Verification items for the finished model (mm, model axes). Face numbers are marked on the shaded views. A direction names the side the tool comes from. Coordinates: 2 decimals unless noted, no trailing zeros. Write each loop counter-clockwise with the first axis right and the second up, starting at its lowest first coordinate (ties: lowest second). Pieces come first, ordered by that corner, then holes. Notation, with made-up numbers: (19, 11) -> (48, 11) arc R23 cw to (48, 29) -> close; hole circle Ø4 at (-5.5, 72.25). An arc over 180 degrees is marked (long way). Answer in a Markdown table with one row per item.
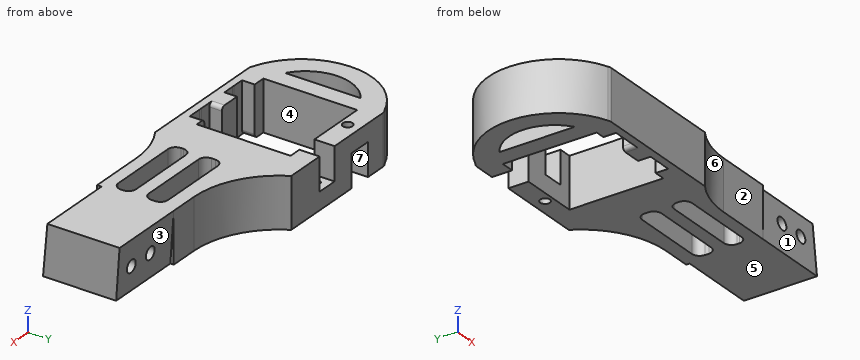
```python
from build123d import *

# Parameters (mm, degrees)
SKETCH_1_W           = 32.6
SKETCH_1_H           = 34.6
SKETCH_1_R           = 1.25
SKETCH_1_W_2         = 24.6
SKETCH_1_H_2         = 24.2
EXTRUDE_1_DEPTH      = 13
SKETCH_3_W           = 6.5
SKETCH_3_H           = 6.519005167
CUT_EXTRUDE_1_DEPTH  = 19
SKETCH_4_W           = 6.5
SKETCH_4_H           = 6.467668889
CUT_EXTRUDE_2_DEPTH  = 23
EXTRUDE_2_DEPTH      = 50
SKETCH_1_2_W         = 22.27659965
SKETCH_1_2_H         = 4.598586669
SKETCH_1_2_W_2       = 22.283050596
SKETCH_1_2_H_2       = 4.977540741
CUT_EXTRUDE_5_DEPTH  = 34
FILLET_1_R           = 2
FILLET_2_R           = 2
FILLET_5_R           = 1
SKETCH_9_W           = 54.594998093
SKETCH_9_H           = 18.111982385
SKETCH_9_W_2         = 52.534809486
SKETCH_9_H_2         = 12.989301534
CUT_EXTRUDE_6_DEPTH  = 41
FILLET_6_R           = 22
EXTRUDE_4_DEPTH      = 13
SKETCH_13_W          = 5.518907879
SKETCH_13_H          = 8.361822047
CUT_EXTRUDE_8_DEPTH  = 8.5
SKETCH_14_W          = 6.038657432
SKETCH_14_H          = 7.741248121
CUT_EXTRUDE_9_DEPTH  = 8.5
SKETCH_15_OUTSIDE_W  = 35.102
SKETCH_15_OUTSIDE_H  = 56.702
CUT_EXTRUDE_11_DEPTH = 20
SKETCH_20_R          = 1.625
CUT_EXTRUDE_15_DEPTH = 40


with BuildPart() as part:
    # Sketch 1 → 凸台-拉伸1 (new body)
    with BuildSketch(Plane.XY):
        with Locations((-9.850980392, 1.274712581)):
            Rectangle(SKETCH_1_W, SKETCH_1_H)
        with Locations(Location((-15.700980392, 15.424712581, 0), (0, 0, 180))):
            Circle(SKETCH_1_R, mode=Mode.SUBTRACT)
        with Locations(Location((-3.600980392, 15.424712581, 0), (0, 0, 180))):
            Circle(SKETCH_1_R, mode=Mode.SUBTRACT)
        with Locations(Location((-15.700980392, -12.875287419, 0), (0, 0, 180))):
            Circle(SKETCH_1_R, mode=Mode.SUBTRACT)
        with Locations(Location((-3.600980392, -12.875287419, 0), (0, 0, 180))):
            Circle(SKETCH_1_R, mode=Mode.SUBTRACT)
        with Locations((-9.850980392, 1.274712581)):
            Rectangle(SKETCH_1_W_2, SKETCH_1_H_2, mode=Mode.SUBTRACT)
    extrude(amount=EXTRUDE_1_DEPTH)

    # 草图3 → 切除-拉伸1 (cut)
    with BuildSketch(Plane(origin=(0, 0, 0), x_dir=(-1, 0, 0), z_dir=(0, 0, -1))):
        with Locations((15.700980392, -10.82528742)):
            Rectangle(SKETCH_3_W, SKETCH_3_H)
    extrude(amount=-CUT_EXTRUDE_1_DEPTH, mode=Mode.SUBTRACT)

    # 草图4 → 切除-拉伸2 (cut)
    with BuildSketch(Plane.XY.offset(13)):
        with Locations((-3.600980392, -10.82528742)):
            Rectangle(SKETCH_4_W, SKETCH_4_H)
    extrude(amount=-CUT_EXTRUDE_2_DEPTH, mode=Mode.SUBTRACT)

    # 草图5 → 凸台-拉伸2 (add)
    with BuildSketch(Plane(origin=(6.449019608, 0, 0), x_dir=(0, 0, -1), z_dir=(1, 0, 0))):
        Polygon((-13, 18.574712581), (-13, 10.055461473), (-13, -16.025287419), (0, -16.025287419), (0, -15.027567927), (0, 16.282461831), (0, 18.574712581), align=None)
    extrude(amount=EXTRUDE_2_DEPTH)

    # Sketch 1 2 → 切除-拉伸5 (cut)
    with BuildSketch(Plane.XY.offset(13)):
        with Locations((24.037173058, -7.263594431)):
            Rectangle(SKETCH_1_2_W, SKETCH_1_2_H)
        with Locations((24.078382453, 0.81654228)):
            Rectangle(SKETCH_1_2_W_2, SKETCH_1_2_H_2)
    extrude(amount=-CUT_EXTRUDE_5_DEPTH, mode=Mode.SUBTRACT)

    # 圆角1
    fillet_1_edges = [part.edges().sort_by_distance(p)[0] for p in [
        (12.936857155, -1.672228091, 6.5),
        (12.936857155, 3.30531265, 6.5),
        (35.219907751, 3.30531265, 6.5),
        (35.219907751, -1.672228091, 6.5),
        (12.898873233, -9.562887765, 6.5),
        (12.898873233, -4.964301096, 6.5),
        (35.175472883, -4.964301096, 6.5),
        (35.175472883, -9.562887765, 6.5),
    ]]
    fillet(fillet_1_edges, radius=FILLET_1_R)

    # 圆角2
    fillet_2_edges = [part.edges().sort_by_distance(p)[0] for p in [
        (-26.150980392, -16.025287419, 6.5),
        (-26.150980392, 18.574712581, 6.5),
    ]]
    fillet(fillet_2_edges, radius=FILLET_2_R)

    # 圆角5
    fillet_5_edges = [part.edges().sort_by_distance(p)[0] for p in [
        (-12.450980392, -12.455038711, 0),
        (-18.950980392, -12.455038711, 0),
        (-6.850980392, -12.442204642, 13),
        (-0.350980392, -12.442204642, 13),
    ]]
    fillet(fillet_5_edges, radius=FILLET_5_R)

    # 草图9 → 切除-拉伸6 (cut)
    with BuildSketch(Plane(origin=(0, 0, 0), x_dir=(-1, 0, 0), z_dir=(0, 0, -1))):
        with Locations((-36.934177516, 16.051357777)):
            Rectangle(SKETCH_9_W, SKETCH_9_H)
        with Locations((-36.653242706, -19.247200889)):
            Rectangle(SKETCH_9_W_2, SKETCH_9_H_2)
    extrude(amount=-CUT_EXTRUDE_6_DEPTH, mode=Mode.SUBTRACT)

    # 圆角6
    # the kernel refuses this fillet: 22 mm, written as the material it adds along each edge
    with BuildSketch(Plane(origin=(9.636678469, 6.995366584, 0), x_dir=(0, 1, 0), z_dir=(0, 0, 1))) as fillet_6_piece_1:
        with BuildLine():
            CenterArc((22, -19.375499223), FILLET_6_R, 118.272534833, 61.727465167)
            Line((0, -19.375499223), (-0.44, -19.375499223))
            Line((-0.44, -19.375499223), (-0.44, 0))
            Line((-0.44, 0), (0, 0.44))
            ThreePointArc((0, 0.44), (5.789672998, 0.44), (11.370932916, 0.387509984))
            Line((11.370932916, 0.387509984), (11.579345996, 0))
        make_face()
    extrude(amount=13)
    with BuildSketch(Plane(origin=(10.385837963, -12.752550122, 0), x_dir=(1, 0, 0), z_dir=(0, 0, 1))) as fillet_6_piece_2:
        with BuildLine():
            CenterArc((11.54511289, -22), FILLET_6_R, 90, 31.653290012)
            Line((0, -3.272737297), (-0.230902258, -2.898192043))
            ThreePointArc((-0.230902258, -2.898192043), (-0.44, -1.636368649), (-0.44, 0))
            Line((-0.44, 0), (0, 0.44))
            Line((0, 0.44), (11.54511289, 0.44))
            Line((11.54511289, 0.44), (11.54511289, 0))
        make_face()
    extrude(amount=13)

    # 草图12 → 凸台-拉伸4 (add)
    with BuildSketch(Plane(origin=(0, 0, 0), x_dir=(-1, 0, 0), z_dir=(0, 0, -1))):
        with BuildLine():
            Line((24.150980392, 18.574712581), (24.496655084, -15.99518818))
            ThreePointArc((24.496655084, -15.99518818), (37.015647173, 1.416671567), (24.150980392, 18.574712581))
        make_face()
        with BuildLine():
            Line((26.822698684, 1.289948959), (26.822698684, -8.431688638))
            ThreePointArc((26.822698684, -8.431688638), (32.027920461, 1.289948959), (26.822698684, 11.011586556))
            Line((26.822698684, 11.011586556), (26.822698684, 1.289948959))
        make_face(mode=Mode.SUBTRACT)
    extrude(amount=-EXTRUDE_4_DEPTH)

    # 草图13 → 切除-拉伸8 (cut)
    with BuildSketch(Plane.XY.offset(13)):
        with Locations((-3.600980393, 15.424712581)):
            Rectangle(SKETCH_13_W, SKETCH_13_H)
    extrude(amount=-CUT_EXTRUDE_8_DEPTH, mode=Mode.SUBTRACT)

    # 草图14 → 切除-拉伸9 (cut)
    with BuildSketch(Plane(origin=(0, 0, 0), x_dir=(-1, 0, 0), z_dir=(0, 0, -1))):
        with Locations((15.700980392, 15.424712581)):
            Rectangle(SKETCH_14_W, SKETCH_14_H)
    extrude(amount=-CUT_EXTRUDE_9_DEPTH, mode=Mode.SUBTRACT)

    # 草图15 outside → 切除-拉伸11 (cut)
    with BuildSketch(Plane(origin=(56.449019608, 0, 0), x_dir=(0, 0, -1), z_dir=(1, 0, 0))):
        with Locations((-6.5, 1.275)):
            Rectangle(SKETCH_15_OUTSIDE_W, SKETCH_15_OUTSIDE_H)
        Polygon((-13, 6.995366584), (6.023241537, 5.707746072), (0, -12.752550122), (-13, -11.615197497), align=None, mode=Mode.SUBTRACT)
    extrude(amount=-CUT_EXTRUDE_11_DEPTH, mode=Mode.SUBTRACT)

    # 草图20 → 切除-拉伸15 (cut)
    with BuildSketch(Plane(origin=(0, 6.087549391, -0.412046152), x_dir=(1, 0, 0), z_dir=(0, 0.9977170964112915, -0.06753218142946318))):
        with Locations(Location((44.449019608, -6.662988966, 0), (0, 0, 270))):
            Circle(SKETCH_20_R)
        with Locations(Location((51.449019608, -6.662988966, 0), (0, 0, 270))):
            Circle(SKETCH_20_R)
    extrude(amount=-CUT_EXTRUDE_15_DEPTH, mode=Mode.SUBTRACT)


solid = part.part
```
1. Depth check by flat-ended pin: P1, Ø0.7, axis at y = -7, z = 6.5, coming from the -X side; P2, Ø4, axis at y = 15, z = 5.5, coming from the -X side; P3, Ø2.5, axis at y = 14.5, z = 8.5, coming from the +X side; P4, Ø2, axis at x = -3.6, y = 15.42, coming from the +Z side (3 decimals). Enter the tip coordinate at first touch or a pass-through.
Geometry says:
| item | result |
|---|---|
| P1 | x = -35.21 |
| P2 | x = -32.68 |
| P3 | x = 13.65 |
| P4 | through |
2. Section check A-A, the plane y = 8.5. Record the boundary of the cut face in (x, z), plus the area to 3 significant figures.
Geometry says:
| item | result |
|---|---|
| outline | (-35.5, 0) -> (-29.54, 0) -> (-29.54, 13) -> (-35.5, 13) -> close; (-26.82, 0) -> (-22.15, 0) -> (-22.15, 13) -> (-26.82, 13) -> close; (2.45, 0) -> (21.02, 0) -> (21.02, 13) -> (2.45, 13) -> close |
| area | 380 mm^2 |
3. Mould release check, pull along X, two halves, no side actions. Record for the marked faces 5, 6 and 7: released by +X, released by -X, zero draft, split by the parting line, or undercut.
Geometry says:
| item | result |
|---|---|
| face 5 | zero draft |
| face 6 | released by +X |
| face 7 | undercut |
4. Tool access check on the marked faces 1, 2, 3 and 4. Record the directions out of +Z, -Z, +X, -X, +Y, -Y that give a thin tool (end or side, any length) a straight path to the whole face; none if there is none.
Geometry says:
| item | result |
|---|---|
| face 1 | +Z, +X, -Y |
| face 2 | +Z, -Z, +X, -Y |
| face 3 | -Z, +X, +Y |
| face 4 | +Z, -Z |
5. Section check B-B, the plane y = -0.5. State how many separate pieces and enclosed holes the cut face has, plus the area to 3 significant figures.
Geometry says:
| item | result |
|---|---|
| separate pieces | 4 |
| enclosed holes | 2 |
| area | 527 mm^2 |
6. Thickness scan on line 1 (X direction, y = -7, z = 7.5); line 2 (Y direction, x = 16, z = 10.25); line 3 (X direction, y = 10, z = 8.5). Record the ranges inside material, lowest first. Write a range as from..to.
Geometry says:
| item | result |
|---|---|
| line 1 | -35.04..-28.58, -26.82..-22.15, 2.45..12.9, 35.18..42.86, 46.04..49.86, 53.04..56.45 |
| line 2 | -13.57..-9.56, -4.96..-1.67, 3.31..11.26 |
| line 3 | -34.76..-28.13, -26.82..-22.15, 2.45..17.91 |
